from build123d import *

# Parameters (mm, degrees)
BOSS_EXTRUDE1_DEPTH = 5.715
BOSS_EXTRUDE2_DEPTH = 6.6675
BOSS_EXTRUDE3_START = 6.6675
BOSS_EXTRUDE3_DEPTH = 6.6675
FILLET1_R           = 2.54
SKETCH5_R           = 1.524
CUT_EXTRUDE1_DEPTH  = 6.35
CUT_EXTRUDE2_DEPTH  = 110.257060148


with BuildPart() as part:
    # Sketch1 → Boss-Extrude1 (new body)
    with BuildSketch(Plane.XY):
        with BuildLine():
            ThreePointArc((69.342, 76.073), (0, 6.731), (-69.342, 76.073))
            Line((-69.342, 76.073), (-76.073, 76.073))
            ThreePointArc((-76.073, 76.073), (0, 0), (76.073, 76.073))
            Line((76.073, 76.073), (69.342, 76.073))
        make_face()
    extrude(amount=BOSS_EXTRUDE1_DEPTH)

    # Sketch3 → Boss-Extrude2 (add)
    with BuildSketch(Plane.XY.offset(5.715)):
        with BuildLine():
            ThreePointArc((65.5955, 76.073), (0, 10.4775), (-65.5955, 76.073))
            Line((-65.5955, 76.073), (-69.342, 76.073))
            ThreePointArc((-69.342, 76.073), (0, 6.731), (69.342, 76.073))
            Line((69.342, 76.073), (65.5955, 76.073))
        make_face()
        with BuildLine():
            Line((76.073, 76.073), (69.342, 76.073))
            ThreePointArc((69.342, 76.073), (0, 6.731), (-69.342, 76.073))
            Line((-69.342, 76.073), (-76.073, 76.073))
            ThreePointArc((-76.073, 76.073), (0, 0), (76.073, 76.073))
        make_face()
    extrude(amount=BOSS_EXTRUDE2_DEPTH)

    # Sketch4 → Boss-Extrude3 (add)
    with BuildSketch(Plane(origin=(0, 0, 0), x_dir=(-1, 0, 0), z_dir=(0, 0, -1)).offset(BOSS_EXTRUDE3_START)):
        with BuildLine():
            ThreePointArc((65.5955, 76.073), (0, 10.4775), (-65.5955, 76.073))
            Line((-65.5955, 76.073), (-69.342, 76.073))
            ThreePointArc((-69.342, 76.073), (0, 6.731), (69.342, 76.073))
            Line((69.342, 76.073), (65.5955, 76.073))
        make_face()
        with BuildLine():
            Line((76.073, 76.073), (69.342, 76.073))
            ThreePointArc((69.342, 76.073), (0, 6.731), (-69.342, 76.073))
            Line((-69.342, 76.073), (-76.073, 76.073))
            ThreePointArc((-76.073, 76.073), (0, 0), (76.073, 76.073))
        make_face()
    extrude(amount=-BOSS_EXTRUDE3_DEPTH)

    # Fillet1
    fillet1_edges = [part.edges().sort_by_distance(p)[0] for p in [
        (0, 6.731, 5.715),
        (0, 6.731, 0),
    ]]
    fillet(fillet1_edges, radius=FILLET1_R)

    # Sketch5 → Cut-Extrude1 (cut)
    with BuildSketch(Plane(origin=(0, 0, 0), x_dir=(1, 0, 0), z_dir=(0, 1, 0))):
        with Locations(Location((0, -2.8575, 0), (0, 0, 90))):
            Circle(SKETCH5_R)
    extrude(amount=CUT_EXTRUDE1_DEPTH, mode=Mode.SUBTRACT)

    # Sketch6 → Cut-Extrude2 (cut, through all)
    with BuildSketch(Plane.XY.offset(12.3825)):
        with BuildLine():
            ThreePointArc((-76.073, 76.073), (-75.604028212, 67.639006454), (-74.202895045, 59.309))
            Line((-74.202895045, 59.309), (-63.417173733, 59.309))
            ThreePointArc((-63.417173733, 59.309), (-65.048638878, 67.620532885), (-65.5955, 76.073))
            Line((-65.5955, 76.073), (-76.073, 76.073))
        make_face()
        with BuildLine():
            ThreePointArc((74.202895045, 59.309), (75.604028212, 67.639006454), (76.073, 76.073))
            Line((76.073, 76.073), (65.5955, 76.073))
            ThreePointArc((65.5955, 76.073), (65.048638878, 67.620532885), (63.417173733, 59.309))
            Line((63.417173733, 59.309), (74.202895045, 59.309))
        make_face()
    extrude(amount=-CUT_EXTRUDE2_DEPTH, mode=Mode.SUBTRACT)


solid = part.part
The model under review builds one solid part; all positions refer to its coordinate system, in mm. A direction names the side the tool comes from. Coordinates: 2 decimals unless noted, no trailing zeros. Write each loop counter-clockwise with the first axis right and the second up, starting at its lowest first coordinate (ties: lowest second). Pieces come first, ordered by that corner, then holes. Notation, with made-up numbers: (32, -6) - (76, -6) arc R18 ccw to (76, 26) - close; hole circle Ø9 at (16.25, 3.25). An arc over 180 degrees is marked (long way). Answer as a JSON object with one key per item and string values. Group by question number.
1. Machinability: for faces 1 (the face through (0.58, 3.13, 1.45)), 2 (the face through (5, 10, 12.382)), 3 (the face through (1.288, 6.743, 2.853)), which of the approach directions +Z, -Z, +X, -X, +Y, -Y give a long, thin tool a straight path to every point of the face, cutting with its end or side? Answer none if there is none.
2. To check wall thickness, follow probe 1 along X at (y, z) = (41.5, 3.75); probe 2 along X at (y, z) = (21, -1.25); probe 3 along Y at (x, z) = (1, 6). State the ranges of each line that lie inside material, in increasing order.
3. Clearance check with flat-ended pins moving along their axes: pin 1 Ø8 at (x, z) = (-47, 9) entering from -Y; pin 2 Ø4 at (x, z) = (-21, 4.5) entering from -Y; pin 3 Ø6 at (y, z) = (16.5, -1.5) entering from -X. State where each tip first meets the part, or that it passes through.
4. Add section B-B (z = 9.75). Give the boundary of the cut face in (x, y), plus the area to 3 significant figures.
5. Mouldability with a two-part tool opening along X and no side actions: class faces 4 (the face through (-4, 10, 0)), 5 (the face through (1.436, 0.014, 0.607)), 6 (the face through (69, 59.309, 3)) as pulls with the +X half, pulls with the -X half, needs draft (parallel to the pull), parting line crosses it, or undercut.
Findings:
{
 "1": {"face 1": "-Y", "face 2": "+Z, +X, -X, +Y, -Y", "face 3": "+Y"},
 "2": {"probe 1": "-67.76 to -60.03, 60.03 to 67.76", "probe 2": "-52.48 to -35.63, 35.63 to 52.48", "probe 3": "0.01 to 10.49"},
 "3": {"pin 1": "y = 13.32", "pin 2": "y = 2.41", "pin 3": "x = -50.86"},
 "4": {"outline": "(-74.2, 59.31) arc R76.07 ccw to (74.2, 59.31) - (63.42, 59.31) arc R65.6 cw to (-63.42, 59.31) - close", "area": "1,980 mm²"},
 "5": {"face 4": "undercut", "face 5": "parting line crosses it", "face 6": "needs draft"}
}
